The listing builds one solid part. Answer for the finished solid, in the listing's coordinates (mm). A direction names the side the tool comes from. Coordinates: 2 decimals unless noted, no trailing zeros. Write each loop counter-clockwise with the first axis right and the second up, starting at its lowest first coordinate (ties: lowest second). Pieces come first, ordered by that corner, then holes.
from build123d import *

# Parameters (mm, degrees)
F1_DEPTH = 25.4
F2_W     = 12.7
F2_H     = 6.35
F3_DEPTH = 25.4
F5_DEPTH = 25.4


# Not quite as in the source:
# - a feature names something its author has since deleted; it is built from what else it names


with BuildPart() as f1:
    # F0 (on Top) → F1 (new body)
    with BuildSketch(Plane.XY):
        Polygon((-3.81, 0), (0, 0), (0, 2.54), (0, 25.4), (-12.7, 25.4), (-25.4, 25.4), (-25.4, 2.54), (-25.4, 0), (-21.59, 0), align=None)
        with BuildLine():
            ThreePointArc((-6.35, 12.7), (-17.1901280605, 8.2098719395), (-12.7, 19.05))
            ThreePointArc((-12.7, 19.05), (-8.2098719395, 17.1901280605), (-6.35, 12.7))
        make_face(mode=Mode.SUBTRACT)
    extrude(amount=F1_DEPTH)

    # F2 (on face) → F3 (cut)
    with BuildSketch(Plane.XZ):
        with Locations((-12.7, 12.7)):
            Rectangle(F2_W, F2_H)
    extrude(amount=-F3_DEPTH, mode=Mode.SUBTRACT)

    # F4 (on face) → F5 (cut)
    with BuildSketch(Plane.YZ):
        with BuildLine():
            ThreePointArc((3.81, 21.59), (3.4380256121, 22.4880256121), (2.54, 22.86))
            Line((2.54, 22.86), (2.54, 21.59))
            Line((2.54, 21.59), (1.27, 21.59))
            ThreePointArc((1.27, 21.59), (2.54, 20.32), (3.81, 21.59))
        make_face()
        with BuildLine():
            Line((2.54, 21.59), (2.54, 22.86))
            ThreePointArc((2.54, 22.86), (1.6419743879, 22.4880256121), (1.27, 21.59))
            Line((1.27, 21.59), (2.54, 21.59))
        make_face()
        with BuildLine():
            ThreePointArc((3.81, 3.81), (2.54, 5.08), (1.27, 3.81))
            Line((1.27, 3.81), (2.54, 3.81))
            Line((2.54, 3.81), (2.54, 2.54))
            ThreePointArc((2.54, 2.54), (3.4380256121, 2.9119743879), (3.81, 3.81))
        make_face()
        with BuildLine():
            Line((2.54, 3.81), (1.27, 3.81))
            ThreePointArc((1.27, 3.81), (1.6419743879, 2.9119743879), (2.54, 2.54))
            Line((2.54, 2.54), (2.54, 3.81))
        make_face()
    extrude(amount=-F5_DEPTH, mode=Mode.SUBTRACT)


solid = f1.part
Q1. Determine the mould class of faces 3 (the face through (-16, 19, 0)), 4 (the face through (-6.35, 13, 13)), 5 (the face through (-13, 25.4, 7)) for opening direction Z: released by +Z, released by -Z, zero draft, split by the parting line, or undercut.
Answers below:
face 3: released by -Z
face 4: undercut
face 5: zero draft
Q2. The part is cut by section C-C, the plane z = 20.75. Write down the section's boundary in (x, y), then the cut area to 3 significant figures.
Answers below:
outline: (-25.4, 0) - (0, 0) - (0, 1.59) - (-25.4, 1.59) - close; (-25.4, 3.49) - (0, 3.49) - (0, 25.4) - (-25.4, 25.4) - close; hole circle Ø12.7 at (-12.7, 12.7)
area: 470 mm2
Q3. The part is cut by section B-B, the plane x = -5.25. Write down the section's boundary in (y, z), then the cut area to 3 significant figures.
Answers below:
outline: (0, 0) - (25.4, 0) - (25.4, 25.4) - (0, 25.4) - close; hole circle Ø2.54 at (2.54, 3.81); hole circle Ø2.54 at (2.54, 21.59)
area: 635 mm2
Q4. Which of the six approach directions +Z, -Z, +X, -X, +Y, -Y give full straight-line access (tool end or side, diameter ignored) to faces 1 (the face through (-16, 19, 25.4)), 2 (the face through (-13, 22, 15.875))?
Answers below:
face 1: +Z, +X, -X, +Y, -Y
face 2: +Y, -Y
Q5. The part is cut by section D-D, the plane y = 9.5. Write down the section's boundary in (x, z) (3 decimals), then the cut area to 3 significant figures.
Answers below:
outline: (-25.4, 0) - (-18.185, 0) - (-18.185, 9.525) - (-19.05, 9.525) - (-19.05, 15.875) - (-18.185, 15.875) - (-18.185, 25.4) - (-25.4, 25.4) - close; (-7.215, 0) - (0, 0) - (0, 25.4) - (-7.215, 25.4) - (-7.215, 15.875) - (-6.35, 15.875) - (-6.35, 9.525) - (-7.215, 9.525) - close
area: 356 mm2
Q6. The part is cut by section A-A, the plane x = -14. Write down the section's boundary in (y, z) (1 decimal), then the cut area to 3 significant figures.
Answers below:
outline: (0, 0) - (6.5, 0) - (6.5, 9.5) - (0, 9.5) - close; (0, 15.9) - (6.5, 15.9) - (6.5, 25.4) - (0, 25.4) - close; (18.9, 0) - (25.4, 0) - (25.4, 9.5) - (18.9, 9.5) - close; (18.9, 15.9) - (25.4, 15.9) - (25.4, 25.4) - (18.9, 25.4) - close; hole circle Ø2.5 at (2.5, 3.8); hole circle Ø2.5 at (2.5, 21.6)
area: 237 mm2
Q7. Find the intervals of material crossed by probe 1 along Y at (x, z) = (-12.7, 21.5); probe 2 along X at (y, z) = (12.7, 19.25); probe 3 along Y at (x, z) = (-12.7, 4.75), in increasing order.
Answers below:
probe 1: y = 0 to 1.27, 3.81 to 6.35, 19.05 to 25.4
probe 2: x = -25.4 to -19.05, -6.35 to 0
probe 3: y = 0 to 1.69, 3.39 to 6.35, 19.05 to 25.4
